Build history of the part. All positions in model axes, mm. A direction names the side the tool comes from. Give positions to 0.01 mm unless a question says otherwise; leave off trailing zeros. Order: outer loops, then holes, each group sorted by start corner. A loop starts at its lowest first (then second) coordinate and runs counter-clockwise, first axis right, second up. Notation, with made-up numbers: (-17.5, 25.25) - (9.5, 25.25) arc R4 cw to (9.5, 32.25) - close; hole circle Ø10 at (27, -35). An arc over 180 degrees is marked (long way). Use a Markdown table: item, result.
from build123d import *

# Parameters (mm, degrees)
SKETCH003_AS_DRAWN_R                 = 1.5
EXTRUDE005_DEPTH                     = 32
EXTRUDE005_ONTO_SKETCH003_ROLL_ANGLE = 90
EXTRUDE002_DEPTH                     = 27
EXTRUDE003_DEPTH                     = 13
SKETCH_R                             = 3.5
EXTRUDE_DEPTH                        = 4
FILLET_R                             = 3
FILLET001_R                          = 1


with BuildPart() as bracket_cut_extrude:
    # Sketch003 as drawn → Extrude005 (new)
    with BuildSketch(Plane.XY):
        with Locations((29.5, -32)):
            Circle(SKETCH003_AS_DRAWN_R)
        with Locations((44.5, -32)):
            Circle(SKETCH003_AS_DRAWN_R)
        with BuildLine():
            Line((34, -37), (34, -16))
            ThreePointArc((40, -16), (37, -13), (34, -16))
            Line((40, -16), (40, -37))
            Line((34, -37), (40, -37))
        make_face()
        with BuildLine():
            Line((18.5, 0), (18.5, -39))
            Line((18.5, -39), (25, -39))
            Line((25, -39), (25, -15.18958))
            ThreePointArc((25, -15.18958), (24.432523, -7.410613), (22, 0))
            Line((18.5, 0), (22, 0))
        make_face()
    extrude(amount=-EXTRUDE005_DEPTH)


with BuildPart() as bracket_cut_extrude_1:
    # Extrude005 onto Sketch003 roll: moved
    add(bracket_cut_extrude.part.rotate(Axis((0, 0, 0), (1, 0, 0)), EXTRUDE005_ONTO_SKETCH003_ROLL_ANGLE))


with BuildPart() as bracket_cut_extrude_2:
    # Extrude005 onto Sketch003 placement: moved
    add(bracket_cut_extrude_1.part.moved(Location((0, -16, 0))))


with BuildPart() as bracket_cut:
    # Sketch001 → Extrude002 (new body)
    with BuildSketch(Plane.YZ.offset(25)):
        with BuildLine():
            ThreePointArc((3, -26.690906), (0, 4.016), (-3, -26.690906))
            Line((-3, -26.690906), (-3, -36.690906))
            Line((-3, -36.690906), (-1.5, -36.690906))
            Line((-1.5, -36.690906), (-1.5, -25.302828))
            ThreePointArc((1.5, -25.302828), (0, 2.416), (-1.5, -25.302828))
            Line((1.5, -36.690906), (1.5, -25.302828))
            Line((3, -36.690906), (1.5, -36.690906))
            Line((3, -26.690906), (3, -36.690906))
        make_face()
    extrude(amount=EXTRUDE002_DEPTH)


with BuildPart() as bracket_cut_1:
    # Extrude002 placement: moved
    add(bracket_cut.part.moved(Location((-3, 0, 0))))

    # Cut001: cut Bracket_Cut_Extrude
    add(bracket_cut_extrude_2.part, mode=Mode.SUBTRACT)


with BuildPart() as cutout_extrude:
    # Sketch002 → Extrude003 (new body)
    with BuildSketch(Plane.YZ.offset(34.801316)):
        with BuildLine():
            ThreePointArc((9.396876, -1.257504), (0, 2.4), (-9.396876, -1.257504))
            Line((-9.396876, -1.257504), (9.396876, -1.257504))
        make_face()
    extrude(amount=-EXTRUDE003_DEPTH)


with BuildPart() as fusion:
    # Sketch → Extrude (new body)
    with BuildSketch(Plane.XY):
        with BuildLine():
            ThreePointArc((15.198684, 13), (-20, 0), (15.198684, -13))
            ThreePointArc((24.801316, -10), (19.786149, -10.815491), (15.198684, -13))
            Line((34.801316, -10), (24.801316, -10))
            Line((34.801316, 10), (34.801316, -10))
            Line((24.801316, 10), (34.801316, 10))
            ThreePointArc((15.198684, 13), (19.786149, 10.815491), (24.801316, 10))
        make_face()
        Circle(SKETCH_R, mode=Mode.SUBTRACT)
        with BuildLine():
            ThreePointArc((3.797918, 6.202082), (3.797918, 3.797918), (6.202082, 3.797918))
            Line((6.202082, 3.797918), (12.202082, 9.797918))
            ThreePointArc((12.202082, 9.797918), (12.202082, 12.202082), (9.797918, 12.202082))
            Line((3.797918, 6.202082), (9.797918, 12.202082))
        make_face(mode=Mode.SUBTRACT)
        with BuildLine():
            ThreePointArc((-6.202082, 3.797918), (-3.797918, 3.797918), (-3.797918, 6.202082))
            Line((-3.797918, 6.202082), (-9.797918, 12.202082))
            ThreePointArc((-9.797918, 12.202082), (-12.202082, 12.202082), (-12.202082, 9.797918))
            Line((-6.202082, 3.797918), (-12.202082, 9.797918))
        make_face(mode=Mode.SUBTRACT)
        with BuildLine():
            ThreePointArc((-3.797918, -6.202082), (-3.797918, -3.797918), (-6.202082, -3.797918))
            Line((-6.202082, -3.797918), (-12.202082, -9.797918))
            ThreePointArc((-12.202082, -9.797918), (-12.202082, -12.202082), (-9.797918, -12.202082))
            Line((-3.797918, -6.202082), (-9.797918, -12.202082))
        make_face(mode=Mode.SUBTRACT)
        with BuildLine():
            ThreePointArc((6.202082, -3.797918), (3.797918, -3.797918), (3.797918, -6.202082))
            Line((3.797918, -6.202082), (9.797918, -12.202082))
            ThreePointArc((9.797918, -12.202082), (12.202082, -12.202082), (12.202082, -9.797918))
            Line((6.202082, -3.797918), (12.202082, -9.797918))
        make_face(mode=Mode.SUBTRACT)
        with BuildLine():
            Line((-15.198684, 9.643651), (-7.5, 1.944967))
            ThreePointArc((-7.5, -1.944967), (-6.694368, 0), (-7.5, 1.944967))
            Line((-15.198684, -9.643651), (-7.5, -1.944967))
            ThreePointArc((-15.198684, 9.643651), (-18, 0), (-15.198684, -9.643651))
        make_face(mode=Mode.SUBTRACT)
        with BuildLine():
            ThreePointArc((-9.671393, -15.181046), (0, -18), (9.671393, -15.181046))
            Line((9.671393, -15.181046), (1.990347, -7.5))
            ThreePointArc((1.990347, -7.5), (0, -6.675571), (-1.990347, -7.5))
            Line((-9.671393, -15.181046), (-1.990347, -7.5))
        make_face(mode=Mode.SUBTRACT)
        with BuildLine():
            ThreePointArc((9.671393, 15.181046), (0, 18), (-9.671393, 15.181046))
            Line((-9.671393, 15.181046), (-1.990347, 7.5))
            ThreePointArc((-1.990347, 7.5), (0, 6.675571), (1.990347, 7.5))
            Line((9.671393, 15.181046), (1.990347, 7.5))
        make_face(mode=Mode.SUBTRACT)
        with BuildLine():
            Line((7.5, 1.116375), (12.503518, 6.119893))
            ThreePointArc((15.198684, 6.896747), (13.750933, 6.855837), (12.503518, 6.119893))
            Line((15.198684, 6.896747), (18.123646, 6.229964))
            ThreePointArc((20.301316, 3.5), (19.690211, 5.246064), (18.123646, 6.229964))
            Line((20.301316, 3.5), (20.301316, -3.5))
            ThreePointArc((18.123646, -6.229964), (19.690211, -5.246064), (20.301316, -3.5))
            Line((18.123646, -6.229964), (15.198684, -6.896747))
            ThreePointArc((12.503518, -6.119893), (13.750933, -6.855837), (15.198684, -6.896747))
            Line((12.503518, -6.119893), (7.5, -1.116375))
            ThreePointArc((7.5, 1.116375), (7.037582, 0), (7.5, -1.116375))
        make_face(mode=Mode.SUBTRACT)
    extrude(amount=EXTRUDE_DEPTH)

    # Cut: cut Cutout_Extrude
    add(cutout_extrude.part, mode=Mode.SUBTRACT)

    # Fillet
    fillet_edges = [fusion.edges().sort_by_distance(p)[0] for p in [
        (29.801316, -10, 4),
        (29.801316, 10, 4),
    ]]
    fillet(fillet_edges, radius=FILLET_R)

    # Fillet001
    fillet001_edges = [fusion.edges().sort_by_distance(p)[0] for p in [
        (34.801316, 0, 4),
    ]]
    fillet(fillet001_edges, radius=FILLET001_R)

    # Fusion: union Bracket_Cut
    add(bracket_cut_1.part)


solid = fusion.part
1) Slice it at C-C (y = 16.5). Write the cut outline in (x, z), and give its area (3 significant figures).
Computed:
| item | result |
|---|---|
| outline | (-11.3, 0) - (-7.19, 0) - (-7.19, 4) - (-11.3, 4) - close; (7.19, 0) - (11.3, 0) - (11.3, 4) - (7.19, 4) - close |
| area | 32.9 mm² |
2) Slice it at D-D (z = -4). Write the cut outline in (x, y), and give its area (3 significant figures).
Computed:
| item | result |
|---|---|
| outline | (23.56, -13.57) - (49, -13.57) - (49, -11.71) - (23.56, -11.71) - close; (23.56, 11.71) - (49, 11.71) - (49, 13.57) - (23.56, 13.57) - close |
| area | 94.6 mm² |
3) Slice it at B-B (z = -28.5). Write the cut outline in (x, y), and give its area (3 significant figures).
Computed:
| item | result |
|---|---|
| outline | (25, -3) - (34, -3) - (34, -1.5) - (25, -1.5) - close; (25, 1.5) - (34, 1.5) - (34, 3) - (25, 3) - close; (40, -3) - (49, -3) - (49, -1.5) - (40, -1.5) - close; (40, 1.5) - (49, 1.5) - (49, 3) - (40, 3) - close |
| area | 54.0 mm² |
4) Slice it at A-A (x = 29.5). State how many separate pieces and enclosed holes the cut face has, and give its area (3 significant figures).
Computed:
| item | result |
|---|---|
| separate pieces | 3 |
| enclosed holes | 0 |
| area | 183 mm² |
5) Pin check, flat tips, straight feed: P1, Ø2, axis at x = -5, y = -7, coming from the -Z side; P2, Ø12, axis at x = -11.5, z = -4.5, coming from the -Y side; P3, Ø5, axis at x = 29.5, z = -32, coming from the +Y side. Stop position of each tip, or through.
Computed:
| item | result |
|---|---|
| P1 | stops at z = 0 |
| P2 | stops at y = -18.53 |
| P3 | stops at y = 3 |
6) Two-plate mould, pull along Y, no slides. Class faces 1 (the cylindrical face through (38.311, 0.639, 4.003)), 2 (the cylindrical face through (12.175, -12.228, 1.972)), 3 (the cylindrical face through (29.24, -9.1, 3.14)): +Y half, -Y half, draft (parallel to the pull), parting line (faces both ways), or undercut.
Computed:
| item | result |
|---|---|
| face 1 | parting line |
| face 2 | undercut |
| face 3 | -Y half |
7) Tool access for faces 4 (the flat face through (28, -3, -31)), 5 (the flat face through (20.301, 0, 2)), 6 (the flat face through (34.801, 8, 2)), 7 (the cylindrical face through (37, 15, -13)): list every direction of +Z, -Z, +X, -X, +Y, -Y with a clear straight run to the whole face (end or side of a thin tool).
Computed:
| item | result |
|---|---|
| face 4 | -Z, +X, -X, -Y |
| face 5 | +Z, -Z |
| face 6 | +Z, +X, +Y |
| face 7 | -Z, +Y, -Y |
8) Wall check: line 1 (Z direction, x = 29.5, y = -2.6); line 2 (Z direction, x = 44.5, y = -2.6); line 3 (Y direction, x = 30, z = -29). Give the ranges that are in metal, low to high. Write a range as from..to.
Computed:
| item | result |
|---|---|
| line 1 | z = -36.69..-33.5, -30.5..-25.14, 2.15..4 |
| line 2 | z = -36.69..-33.5, -30.5..-25.14, 2.17..3.8 |
| line 3 | y = -3..-1.5, 1.5..3 |
